```python
from build123d import *

# Parameters (mm, degrees)
PAD002_DEPTH      = 410
PAD002_DEPTH_BACK = 170
POCKET_DEPTH      = 5
PAD_DEPTH         = 20
SKETCH004_R       = 8
POCKET001_DEPTH   = 10


with BuildPart() as part:
    # Sketch002 → Pad002 (new body, two sides)
    with BuildSketch(Plane(origin=(0, 0, 0), x_dir=(-1, 0, 0), z_dir=(0, 1, 0))) as pad002_sk:
        Polygon((40, 50), (156.2868487308, 369.4954910672), (207.969942874, 350.6843831843), (91.6830941432, 31.1888921171), align=None)
    extrude(amount=PAD002_DEPTH)
    extrude(pad002_sk.sketch, amount=-PAD002_DEPTH_BACK)

    # Sketch (on Face1 of Pad002) → Pocket (cut)
    with BuildSketch(Plane(origin=(-19.2511986202, 0, -7.0068632717), x_dir=(-0.3420201433, 0, 0.9396926208), z_dir=(0.9396926208, 0, 0.3420201433))):
        Polygon((82.9319106246, 85), (388.9319106246, 85), (388.9319106246, -325), (82.9319106246, -325), (82.9319106246, -120), align=None)
    extrude(amount=-POCKET_DEPTH, mode=Mode.SUBTRACT)

    # Sketch003 (on Face11 of Pocket) → Pad (join)
    with BuildSketch(Plane(origin=(-70.9342927634, 0, -25.8179711546), x_dir=(0.3420201433, 0, -0.9396926208), z_dir=(-0.9396926208, 0, -0.3420201433))):
        Polygon((-366.6654367723, -325), (-94.6654367723, -325), (-94.6654367723, -120), (-94.6654367723, 85), (-366.6654367723, 85), align=None)
    extrude(amount=PAD_DEPTH)

    # Sketch004 (on Face18 of Pad) → Pocket001 (cut)
    with BuildSketch(Plane(origin=(-89.7281451791, 0, -32.6583740211), x_dir=(0.3420201433, 0, -0.9396926208), z_dir=(-0.9396926208, 0, -0.3420201433))):
        with Locations((-235.6654367723, -82.5)):
            Circle(SKETCH004_R)
        with Locations((-160.6654367723, -82.5)):
            Circle(SKETCH004_R)
        with Locations((-160.6654367723, -157.5)):
            Circle(SKETCH004_R)
        with Locations((-235.6654367723, -157.5)):
            Circle(SKETCH004_R)
    extrude(amount=-POCKET001_DEPTH, mode=Mode.SUBTRACT)


solid = part.part
```
Input: part model. Units: mm. Frame: model coordinates. A direction names the side the tool comes from. Coordinates: 2 decimals unless noted, no trailing zeros. Loops run counter-clockwise (first coordinate to the right, second up) from the corner with the lowest first, then second, coordinate; pieces in that order, holes last. Notation, with made-up numbers: M 51.5,-30.5 L 75.5,-30.5 A28 cw 75.5,-4.5 Z; hole C 76,29.5 d9. An arc over 180 degrees is marked long. One line per item, written item: value.
(1) Pin query (flat end, axial travel): pin 1 (1 mm diameter, centred on y = 79, z = 163, fed in from -X); pin 2 (10 mm diameter, centred on y = 342, z = 73, fed in from -X); pin 3 (12 mm diameter, centred on y = 50, z = 282, fed in from -X). Return the tip coordinate at first contact, or that it passes through.
Filled in:
pin 1: x = -161.12
pin 2: x = -108.72
pin 3: x = -206.44
(2) Reachability of faces 4 (the flat face through (-112.577, 122.87, 59.766)), 5 (the flat face through (-66.203, 124.06, 40.463)), 6 (the flat face through (-135.32, 157.39, 121.84)) from +Z, -Z, +X, -X, +Y, -Y: full face, straight path, thin tool, end or side. Return the list, or none.
Filled in:
face 4: -Z, +Y, -Y
face 5: -Z, +X, +Y, -Y
face 6: none
(3) Section C-C (z = 270). Output: boundary loops of the cut face in (x, y).
Filled in:
outline: M -199.89,-85 L -178.6,-85 L -178.6,-170 L -120.07,-170 L -120.07,-85 L -125.39,-85 L -125.39,325 L -120.07,325 L -120.07,410 L -178.6,410 L -178.6,325 L -199.89,325 Z
(4) Section D-D (x = -85.5). Output: boundary loops of the cut face in (y, z), and give its area (3 significant figures).
Filled in:
outline: M -170,33.44 L 410,33.44 L 410,175.01 L 325,175.01 L 325,160.39 L -85,160.39 L -85,175.01 L -170,175.01 Z
area: 76,100 mm^2
(5) Line query: line 1 along Y through (x, z) = (-57.5, 91); line 2 along X through (y, z) = (258, 156.5); line 3 along X through (y, z) = (327.5, 84.5). Output: solid intervals per line, ascending. Write a range as from..to.
Filled in:
line 1: -170..-85, 325..410
line 2: -158.58..-84.08
line 3: -111.09..-52.56
(6) Section A-A (y = 232). Output: boundary loops of the cut face in (x, z), and give its area (3 significant figures).
Filled in:
outline: M -215.14,311.89 L -122.11,56.3 L -103.31,63.14 L -91.68,31.19 L -40,50 L -47.62,70.92 L -52.31,69.21 L -156.97,356.76 L -152.27,358.47 L -156.29,369.5 L -207.97,350.68 L -196.34,318.73 Z
area: 22,600 mm^2
(7) Section B-B (x = -180). Output: boundary loops of the cut face in (y, z).
Filled in:
outline: M -170,273.84 L -85,273.84 L -85,215.36 L 325,215.36 L 325,273.84 L 410,273.84 L 410,360.86 L -170,360.86 Z
(8) Pull-direction query (Y, two-part tool) for faces 1 (the cylindrical face through (-140.402, 74.568, 120.983)), 2 (the flat face through (-124, 410, 189)), 3 (the flat face through (-205.61, 117.13, 315.36)); classes: +Y half, -Y half, draft (parallel to the pull), parting line (faces both ways), or undercut.
Filled in:
face 1: undercut
face 2: +Y half
face 3: draft
